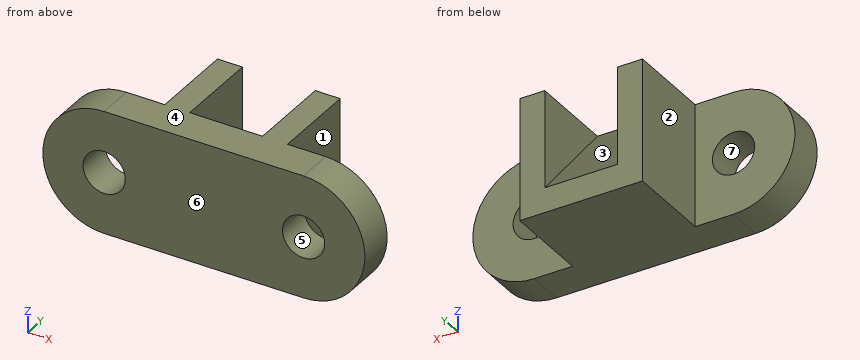
```python
from build123d import *

# Parameters (mm, degrees)
SKETCH_2_R      = 11
EXTRUDE_1_DEPTH = 19
EXTRUDE_2_DEPTH = 45
EXTRUDE_3_DEPTH = 38


with BuildPart() as part:
    # 스케치2 → 보스-돌출1 (new body)
    with BuildSketch(Plane(origin=(0, 0, 0), x_dir=(1, 0, 0), z_dir=(0, 1, 0))):
        with BuildLine():
            Line((0, 0), (104, 0))
            ThreePointArc((104, 0), (136, 32), (104, 64))
            Line((104, 64), (0, 64))
            ThreePointArc((0, 64), (-32, 32), (0, 0))
        make_face()
        with Locations(Location((0, 32, 0), (0, 0, 270))):
            Circle(SKETCH_2_R, mode=Mode.SUBTRACT)
        with Locations(Location((104, 32, 0), (0, 0, 270))):
            Circle(SKETCH_2_R, mode=Mode.SUBTRACT)
    extrude(amount=EXTRUDE_1_DEPTH)

    # 스케치3 → 보스-돌출2 (add)
    with BuildSketch(Plane(origin=(0, 19, 0), x_dir=(1, 0, 0), z_dir=(0, 1, 0))):
        Polygon((84, 0), (84, 64), (20, 64), (20, 0), (33, 0), (33, 51), (71, 51), (71, 0), align=None)
    extrude(amount=EXTRUDE_2_DEPTH)

    # 스케치6 → 보스-돌출3 (add)
    with BuildSketch(Plane(origin=(33, 0, 0), x_dir=(0, 0, -1), z_dir=(1, 0, 0))):
        Polygon((51, 64), (0, 19), (51, 19), align=None)
    extrude(amount=EXTRUDE_3_DEPTH)


solid = part.part
```
Build history of the part. All positions in model axes, mm. Face numbers are marked on the shaded views. A direction names the side the tool comes from. Coordinates: 2 decimals unless noted, no trailing zeros. Order: outer loops, then holes, each group sorted by start corner. A loop starts at its lowest first (then second) coordinate and runs counter-clockwise, first axis right, second up.
Item 1: Mould opens along Z. For the marked faces 4, 5, 6 and 7 say: released by +Z, released by -Z, zero draft, split by the parting line, or undercut.
Filled in:
face 4: released by +Z
face 5: undercut
face 6: zero draft
face 7: undercut
Item 2: Drop flat-ended pins along their axis: pin 1 Ø10 at (x, z) = (-2.5, -51.5) entering from +Y; pin 2 Ø17.5 at (x, z) = (104, -32) entering from +Y; pin 3 Ø4 at (y, z) = (13, -50.5) entering from -X; pin 4 Ø22.5 at (y, z) = (37, -34) entering from +X. Give the stop position or say it passes through.
Filled in:
pin 1: stops at y = 19
pin 2: passes through
pin 3: stops at x = -27.42
pin 4: stops at x = 84
Item 3: Saw through at D-D on y = 13.5. List the corners of the cut face in (x, z), then the cut area to 3 significant figures.
Filled in:
outline: (0, -64) - (104, -64) arc R32 ccw to (104, 0) - (0, 0) arc R32 ccw to start; hole circle Ø22 at (0, -32); hole circle Ø22 at (104, -32)
area: 9,110 mm2
Item 4: Drill centre lines: L1, parallel to X at y = 6, z = -32; L2, parallel to X at y = 60, z = -25; L3, parallel to X at y = 51.5, z = -39. Where is each one in solid material? Low to high.
Filled in:
L1: x = -32 to -11, 11 to 93, 115 to 136
L2: x = 20 to 33, 71 to 84
L3: x = 20 to 84
Item 5: Saw through at A-A on z = -35. List the corners of the cut face in (x, y).
Filled in:
outline: (-31.86, 0) - (-10.58, 0) - (-10.58, 19) - (-31.86, 19) - close; (10.58, 0) - (93.42, 0) - (93.42, 19) - (84, 19) - (84, 64) - (71, 64) - (71, 49.88) - (33, 49.88) - (33, 64) - (20, 64) - (20, 19) - (10.58, 19) - close; (114.58, 0) - (135.86, 0) - (135.86, 19) - (114.58, 19) - close
Item 6: Saw through at C-C on y = 58. List the corners of the cut face in (x, z), then the cut area to 3 significant figures.
Filled in:
outline: (20, -64) - (84, -64) - (84, 0) - (71, 0) - (71, -44.2) - (33, -44.2) - (33, 0) - (20, 0) - close
area: 2,420 mm2
Item 7: Saw through at B-B on x = 8. List the corners of the cut face in (y, z), then the cut area to 3 significant figures.
Filled in:
outline: (0, -64) - (19, -64) - (19, -39.55) - (0, -39.55) - close; (0, -24.45) - (19, -24.45) - (19, 0) - (0, 0) - close
area: 929 mm2
Item 8: Tool access for the marked faces 1, 2 and 3: list every direction of +Z, -Z, +X, -X, +Y, -Y with a clear straight run to the whole face (end or side of a thin tool).
Filled in:
face 1: +Z, -Z, +X, +Y
face 2: +Z, -Z, -X, +Y
face 3: +Z, +Y
